```python
from build123d import *

# Parameters (mm, degrees)
SKETCH1_R           = 15.875
BOSS_EXTRUDE1_DEPTH = 25.4
CUT_EXTRUDE5_START  = -11.49604
SKETCH2_R           = 12.7
CUT_EXTRUDE5_DEPTH  = 11.49604
SKETCH3_R           = 1.7272
CUT_EXTRUDE6_DEPTH  = 26.4
CIRPATTERN3_COUNT   = 4
SKETCH6_R           = 15.875
BOSS_EXTRUDE2_DEPTH = 7.9502
SKETCH7_R           = 2.54
CUT_EXTRUDE7_DEPTH  = 26.4
CHAMFER1_SIZE       = 2.38


with BuildPart() as part:
    # Sketch1 → Boss-Extrude1 (new body)
    with BuildSketch(Plane(origin=(0, 0, 0), x_dir=(1, 0, 0), z_dir=(0, 1, 0))):
        Circle(SKETCH1_R)
    extrude(amount=BOSS_EXTRUDE1_DEPTH)

    # Sketch2 → Cut-Extrude5 (cut)
    with BuildSketch(Plane(origin=(0, 25.4, 0), x_dir=(1, 0, 0), z_dir=(0, 1, 0)).offset(CUT_EXTRUDE5_START)):
        Circle(SKETCH2_R)
    extrude(amount=CUT_EXTRUDE5_DEPTH, mode=Mode.SUBTRACT)

    # Sketch3 → Cut-Extrude6 (cut, through all)
    with BuildSketch(Plane.XZ):
        with Locations((0, 9.525)):
            Circle(SKETCH3_R)
    cut_extrude6 = extrude(amount=-CUT_EXTRUDE6_DEPTH, mode=Mode.SUBTRACT)

    # CirPattern3: Cut-Extrude6 ×4 about axis
    cirpattern3_axis = Axis((0, 0, 0), (0, 1, 0))
    for i in range(1, CIRPATTERN3_COUNT):
        add(cut_extrude6.rotate(cirpattern3_axis, i * 360 / CIRPATTERN3_COUNT), mode=Mode.SUBTRACT)

    # Sketch6 → Boss-Extrude2 (add)
    with BuildSketch(Plane(origin=(0, 25.4, 0), x_dir=(1, 0, 0), z_dir=(0, 1, 0))):
        with BuildLine():
            Line((-63.5, 19.05), (63.5, 19.05))
            ThreePointArc((63.5, 19.05), (82.55, 0), (63.5, -19.05))
            Line((63.5, -19.05), (-63.5, -19.05))
            ThreePointArc((-63.5, -19.05), (-82.55, 0), (-63.5, 19.05))
        make_face()
        Circle(SKETCH6_R, mode=Mode.SUBTRACT)
    extrude(amount=-BOSS_EXTRUDE2_DEPTH)

    # Sketch7 → Cut-Extrude7 (cut, through all)
    with BuildSketch(Plane(origin=(0, 25.4, 0), x_dir=(1, 0, 0), z_dir=(0, 1, 0))):
        with Locations((57.15, 12.7)):
            Circle(SKETCH7_R)
        with Locations((57.15, -12.7)):
            Circle(SKETCH7_R)
        with Locations((-57.15, -12.7)):
            Circle(SKETCH7_R)
        with Locations((-57.15, 12.7)):
            Circle(SKETCH7_R)
    extrude(amount=-CUT_EXTRUDE7_DEPTH, mode=Mode.SUBTRACT)

    # Chamfer1
    chamfer1_edges = [part.edges().sort_by_distance(p)[0] for p in [
        (-15.875, 17.4498, 0),
    ]]
    chamfer(chamfer1_edges, length=CHAMFER1_SIZE)


solid = part.part
```
The model under review builds one solid part; all positions refer to its coordinate system, in mm. A direction names the side the tool comes from. Round coordinates to 2 decimals unless told otherwise and drop trailing zeros. Loops run counter-clockwise (first coordinate to the right, second up) from the corner with the lowest first, then second, coordinate; pieces in that order, holes last. Notation, with made-up numbers: (86, 25) - (142, 25) arc R16 ccw to (142, 36) - close; hole circle Ø1 at (43.5, 41). An arc over 180 degrees is marked (long way). Write each question's results on one line, items separated by ' | '. Start each with the question number.
Q1. Take a section at B-B on y = 20. Give the boundary of the cut face in (x, z).
Q2. Take a section at C-C on x = 57.15. Give the boundary of the cut face in (y, z).
Q3. Tool access review of faces 1 (the cylindrical face through (-1.65, 6.85, -10.04)), 2 (the flat face through (0, 13.904, 0)): name each direction out of +Z, -Z, +X, -X, +Y, -Y from which nothing blocks a thin tool from reaching the whole face with its end or side.
Q4. Insertion check: P1, Ø4.5, axis at x = -9.525, z = 0, coming from the +Y side; P2, Ø8, axis at x = -8, y = 6.5, coming from the -Z side; P3, Ø3, axis at x = 57.15, z = 12.7, coming from the +Y side; P4, Ø3, axis at x = -42, z = 11.5, coming from the -Y side. Each pin has a flat end and moves straight along its axis. Give the tip position at first contact, or say it passes through.
Q5. Take a section at A-A on x = 0. Give the boundary of the cut face in (y, z) (3 decimals).
Q6. Take a section at D-D on y = 10.5. Give the boundary of the cut face in (x, z) (3 decimals).
Q7. Wall thickness on line 1 along Z through (x, y) = (0, 5) (3 decimals); line 2 along Z through (x, y) = (-57.15, 19.5): over which ranges is each line inside the solid? List them lowest first. Write a range as [from, to].
Q8. Draft analysis for pull direction X (two halves, no side actions). For faces 3 (the cylindrical face through (-54.727, 21.481, -13.463)), 4 (the flat face through (-17, 17.45, 8)), 5 (the cylindrical face through (-3.441, 7.429, 15.497)), state which applies: pulls with the +X half, pulls with the -X half, needs draft (parallel to the pull), parting line crosses it, or undercut.
Data:
1) outline: (-63.5, -19.05) - (63.5, -19.05) arc R19.05 ccw to (63.5, 19.05) - (-63.5, 19.05) arc R19.05 ccw to start; hole circle Ø5.08 at (-57.15, -12.7); hole circle Ø5.08 at (-57.15, 12.7); hole circle Ø25.4 at (0, 0); hole circle Ø5.08 at (57.15, -12.7); hole circle Ø5.08 at (57.15, 12.7)
2) outline: (17.45, -19.05) - (25.4, -19.05) - (25.4, -15.24) - (17.45, -15.24) - close; (17.45, -10.16) - (25.4, -10.16) - (25.4, 10.16) - (17.45, 10.16) - close; (17.45, 15.24) - (25.4, 15.24) - (25.4, 19.05) - (17.45, 19.05) - close
3) face 1: +Y, -Y | face 2: +Y
4) P1: stops at y = 13.9 | P2: stops at z = -15.36 | P3: passes through | P4: stops at y = 17.45
5) outline: (0, -15.875) - (15.07, -15.875) - (17.45, -18.255) - (17.45, -19.05) - (25.4, -19.05) - (25.4, -12.7) - (13.904, -12.7) - (13.904, -11.252) - (0, -11.252) - close; (0, -7.798) - (13.904, -7.798) - (13.904, 7.798) - (0, 7.798) - close; (0, 11.252) - (13.904, 11.252) - (13.904, 12.7) - (25.4, 12.7) - (25.4, 19.05) - (17.45, 19.05) - (17.45, 18.255) - (15.07, 15.875) - (0, 15.875) - close
6) outline: circle Ø31.75 at (0, 0); hole circle Ø3.454 at (-9.525, 0); hole circle Ø3.454 at (0, -9.525); hole circle Ø3.454 at (0, 9.525); hole circle Ø3.454 at (9.525, 0)
7) line 1: z = [-15.875, -11.252], [-7.798, 7.798], [11.252, 15.875] | line 2: z = [-19.05, -15.24], [-10.16, 10.16], [15.24, 19.05]
8) face 3: undercut | face 4: needs draft | face 5: parting line crosses it
